Input: part model. Units: mm. Frame: model coordinates. Round coordinates to 2 decimals unless told otherwise and drop trailing zeros. Order: outer loops, then holes, each group sorted by start corner. A loop starts at its lowest first (then second) coordinate and runs counter-clockwise, first axis right, second up. Notation, with made-up numbers: (19.5, 35.25) -> (27.5, 35.25) arc R15 ccw to (27.5, 51.25) -> close; hole circle Ø6 at (57, -16.5). An arc over 180 degrees is marked (long way). Use a Markdown table: item, result.
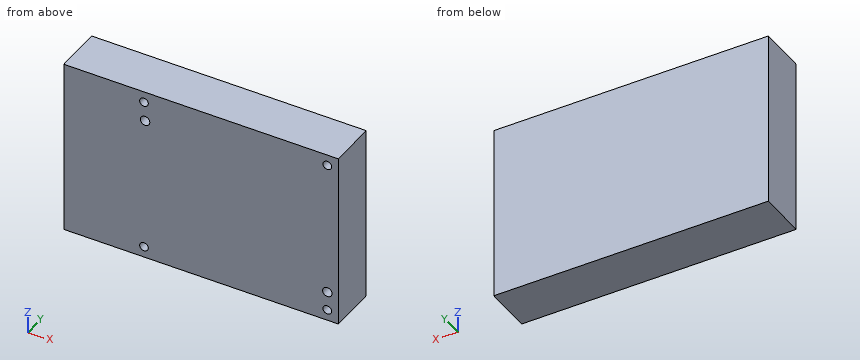
from build123d import *

# Parameters (mm, degrees)
SKETCH_1_W          = 87
SKETCH_1_H          = 56
EXTRUDE_1_DEPTH     = 15.15
SKETCH_2_R          = 1.364499713
SKETCH_2_R_2        = 1.5
CUT_EXTRUDE_1_DEPTH = 10


with BuildPart() as part:
    # Эскиз1 → Бобышка-Вытянуть1 (new body)
    with BuildSketch(Plane(origin=(0, 0, 0), x_dir=(1, 0, 0), z_dir=(0, 1, 0))):
        Rectangle(SKETCH_1_W, SKETCH_1_H)
    extrude(amount=EXTRUDE_1_DEPTH)

    # Эскиз2 → Вырез-Вытянуть1 (cut)
    with BuildSketch(Plane.XZ):
        with Locations(Location((40, 24.5, 0), (0, 0, 270))):
            Circle(SKETCH_2_R)
        with Locations(Location((40.032744033, -18.451055431, 0), (0, 0, 270))):
            Circle(SKETCH_2_R_2)
        with Locations(Location((40, -24.5, 0), (0, 0, 270))):
            Circle(SKETCH_2_R)
        with Locations(Location((-18.085512482, -24.5, 0), (0, 0, 270))):
            Circle(SKETCH_2_R)
        with Locations(Location((-17.736958402, 18.300913925, 0), (0, 0, 270))):
            Circle(SKETCH_2_R_2)
        with Locations(Location((-18.085512482, 24.5, 0), (0, 0, 270))):
            Circle(SKETCH_2_R)
    extrude(amount=-CUT_EXTRUDE_1_DEPTH, mode=Mode.SUBTRACT)


solid = part.part
1) Cut plane A-A on z = -24.5. Return loops of the section in (x, y).
Results found:
| item | result |
|---|---|
| outline | (-43.5, 0) -> (-19.45, 0) -> (-19.45, 10) -> (-16.72, 10) -> (-16.72, 0) -> (38.64, 0) -> (38.64, 10) -> (41.36, 10) -> (41.36, 0) -> (43.5, 0) -> (43.5, 15.15) -> (-43.5, 15.15) -> close |
2) Pin query (flat end, axial travel): pin 1 Ø0.8 at (x, z) = (39.5, 24.5) entering from -Y. Return the tip coordinate at first contact, or that it passes through.
Results found:
| item | result |
|---|---|
| pin 1 | stops at y = 10 |
3) Cut plane B-B on z = 18. Return loops of the section in (x, y).
Results found:
| item | result |
|---|---|
| outline | (-43.5, 0) -> (-19.21, 0) -> (-19.21, 10) -> (-16.27, 10) -> (-16.27, 0) -> (43.5, 0) -> (43.5, 15.15) -> (-43.5, 15.15) -> close |
4) Line query: L1, parallel to X at y = 6.75, z = 24.5; L2, parallel to Z at x = -18.5, y = 6.25; L3, parallel to Z at x = -19, y = 3.75. Output: solid intervals per line, ascending. Write a range as [from, to].
Results found:
| item | result |
|---|---|
| L1 | x = [-43.5, -19.45], [-16.72, 38.64], [41.36, 43.5] |
| L2 | z = [-28, -25.8], [-23.2, 17.01], [19.59, 23.2], [25.8, 28] |
| L3 | z = [-28, -25.51], [-23.49, 17.49], [19.11, 23.49], [25.51, 28] |
